```python
from build123d import *

# Parameters (mm, degrees)
F0_W     = 45
F0_H     = 250
F1_DEPTH = 2.3
F3_D     = 6.6
F4_SIZE  = 3


with BuildPart() as f1:
    # F0 (on Top) → F1 (new body)
    with BuildSketch(Plane.XY):
        with Locations((22.5, 125)):
            Rectangle(F0_W, F0_H)
    extrude(amount=F1_DEPTH)

    # F3 (through all)
    with Locations(Plane.XY.offset(2.3)):
        with Locations((30, 230), (10, 125), (30, 20)):
            Hole(F3_D / 2)

    # F4
    f4_edges = [f1.edges().sort_by_distance(p)[0] for p in [
        (0, 250, 1.15),
        (45, 250, 1.15),
        (0, 0, 1.15),
        (45, 0, 1.15),
    ]]
    chamfer(f4_edges, length=F4_SIZE)


solid = f1.part
```
Verification items for the finished model (mm, model axes). Round coordinates to 2 decimals unless told otherwise and drop trailing zeros. Order: outer loops, then holes, each group sorted by start corner. A loop starts at its lowest first (then second) coordinate and runs counter-clockwise, first axis right, second up. Notation, with made-up numbers: (60, 23) -> (93, 23) arc R23 cw to (93, 62) -> close; hole circle Ø4 at (19, 7). An arc over 180 degrees is marked (long way). Put each result on its own line as item: value. Start each with the question number.
(1) Material ranges on line 1 along Y through (x, z) = (30, 0.55); line 2 along Y through (x, z) = (10, 0.9); line 3 along Y through (x, z) = (33, 1.95), recorded low to high.
(2) Draft check along X on faces 1 (the face through (26.95, 18.74, 1.13)), 2 (the face through (22, 127, 2.3)). Enter one of: +X half, -X half, draft (parallel to the pull), parting line (faces both ways), or undercut.
(3) Depth check by flat-ended pin: pin 1 Ø10.5 at (x, y) = (30, 20) entering from -Z. Enter the tip coordinate at first touch or a pass-through.
(4) Section check B-B (x = 30). Enter the section's corners in (y, z).
(5) Section check C-C (x = 10). Enter the section's corners in (y, z), then the cut area to 3 significant figures.
(6) Section check A-A (y = 230). Enter the section's corners in (x, z), then the cut area to 3 significant figures.
Completed:
1. line 1: y = 0 to 16.7, 23.3 to 226.7, 233.3 to 250
1. line 2: y = 0 to 121.7, 128.3 to 250
1. line 3: y = 0 to 18.63, 21.37 to 228.63, 231.37 to 250
2. face 1: undercut
2. face 2: draft
3. pin 1: stops at z = 0
4. outline: (0, 0) -> (16.7, 0) -> (16.7, 2.3) -> (0, 2.3) -> close; (23.3, 0) -> (226.7, 0) -> (226.7, 2.3) -> (23.3, 2.3) -> close; (233.3, 0) -> (250, 0) -> (250, 2.3) -> (233.3, 2.3) -> close
5. outline: (0, 0) -> (121.7, 0) -> (121.7, 2.3) -> (0, 2.3) -> close; (128.3, 0) -> (250, 0) -> (250, 2.3) -> (128.3, 2.3) -> close
5. area: 560 mm2
6. outline: (0, 0) -> (26.7, 0) -> (26.7, 2.3) -> (0, 2.3) -> close; (33.3, 0) -> (45, 0) -> (45, 2.3) -> (33.3, 2.3) -> close
6. area: 88.3 mm2
